Design review of the part built by this model. Coordinates are the model's own, in mm. Coordinates: 2 decimals unless noted, no trailing zeros. Loops run counter-clockwise (first coordinate to the right, second up) from the corner with the lowest first, then second, coordinate; pieces in that order, holes last. Notation, with made-up numbers: (-36.5, -17) -> (0.5, -17) arc R25 cw to (0.5, 12) -> close; hole circle Ø1 at (8, 47.25). An arc over 180 degrees is marked (long way). Use a Markdown table: item, result. Add a question column.
Q1. For probe 1 along X at (y, z) = (91.5, 2.35); probe 2 along Y at (x, z) = (-109, 0.55); probe 3 along Y at (x, z) = (-103, 1.65), list the stretches that pass through material, from the lowest coordinate up.
Q2. Clearance check with flat-ended pins moving along their axes: pin 1 Ø1 at (x, z) = (-113, 1) entering from +Y; pin 2 Ø10 at (x, y) = (-103.64, 86.83) entering from +Z. State where each tip first meets the part, or that it passes through.
Q3. Take a section at B-B on z = 2.9. Write out the cut boundary in (x, y).
Q4. Take a section at C-C on x = -103.5. Write out the cut boundary in (y, z).
Q5. Take a section at A-A on y = 91. Write out the cut boundary in (x, z).
Q6. Take a section at D-D on y = 81. Write out the cut boundary in (x, z).
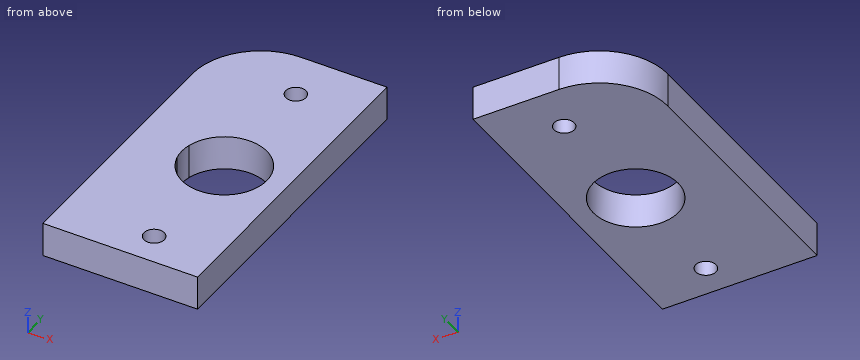
from build123d import *

# Parameters (mm, degrees)
SKETCH1_R           = 1.5
SKETCH1_R_2         = 1.517913389
BOSS_EXTRUDE1_DEPTH = 5.08


with BuildPart() as part:
    # Sketch1 → Boss-Extrude1 (new body)
    with BuildSketch(Plane(origin=(0, 0, 0), x_dir=(-1, 0, 0), z_dir=(0, 0, 1))):
        with BuildLine():
            Line((94.361674585, -111.794978321), (94.361674585, -64.328592097))
            Line((94.361674585, -64.328592097), (117.281412131, -64.328592097))
            Line((117.281412131, -64.328592097), (117.281412131, -101.902374013))
            ThreePointArc((117.281412131, -101.902374013), (114.305617027, -109.08657891), (107.121412131, -112.062374013))
            Line((107.121412131, -112.062374013), (94.361674585, -112.062374013))
            Line((94.361674585, -112.062374013), (94.361674585, -111.794978321))
        make_face()
        with Locations(Location((103.635582515, -104.844491412, 0), (0, 0, 180))):
            Circle(SKETCH1_R, mode=Mode.SUBTRACT)
        with Locations(Location((103.635582515, -69.140487693, 0), (0, 0, 180))):
            Circle(SKETCH1_R_2, mode=Mode.SUBTRACT)
        with BuildLine():
            ThreePointArc((109.76359006, -85.328738191), (97.326662127, -86.828738191), (109.76359006, -88.328738191))
            ThreePointArc((109.76359006, -88.328738191), (109.944502904, -86.828738191), (109.76359006, -85.328738191))
        make_face(mode=Mode.SUBTRACT)
    extrude(amount=BOSS_EXTRUDE1_DEPTH)


solid = part.part
Answer list:
| question | item | result |
|---|---|---|
| 1 | probe 1 | -117.28 to -107.88, -99.4 to -94.36 |
| 1 | probe 2 | 64.33 to 83.51, 90.15 to 111.89 |
| 1 | probe 3 | 64.33 to 67.76, 70.52 to 80.55, 93.11 to 103.49, 106.2 to 112.06 |
| 2 | pin 1 | y = 110.52 |
| 2 | pin 2 | through |
| 3 | outline | (-117.28, 64.33) -> (-94.36, 64.33) -> (-94.36, 112.06) -> (-107.12, 112.06) arc R10.16 ccw to (-117.28, 101.9) -> close; hole circle Ø12.62 at (-103.64, 86.83); hole circle Ø3.04 at (-103.64, 69.14); hole circle Ø3 at (-103.64, 104.84) |
| 4 | outline | (64.33, 0) -> (67.63, 0) -> (67.63, 5.08) -> (64.33, 5.08) -> close; (70.65, 0) -> (80.52, 0) -> (80.52, 5.08) -> (70.65, 5.08) -> close; (93.14, 0) -> (103.35, 0) -> (103.35, 5.08) -> (93.14, 5.08) -> close; (106.34, 0) -> (112.06, 0) -> (112.06, 5.08) -> (106.34, 5.08) -> close |
| 5 | outline | (-117.28, 0) -> (-108.37, 0) -> (-108.37, 5.08) -> (-117.28, 5.08) -> close; (-98.9, 0) -> (-94.36, 0) -> (-94.36, 5.08) -> (-98.9, 5.08) -> close |
| 6 | outline | (-117.28, 0) -> (-106.05, 0) -> (-106.05, 5.08) -> (-117.28, 5.08) -> close; (-101.22, 0) -> (-94.36, 0) -> (-94.36, 5.08) -> (-101.22, 5.08) -> close |
